Geometry check sheet. Reference: the model listing, model coordinates, mm. A direction names the side the tool comes from. Coordinates: 2 decimals unless noted, no trailing zeros. Write each loop counter-clockwise with the first axis right and the second up, starting at its lowest first coordinate (ties: lowest second). Pieces come first, ordered by that corner, then holes.
from build123d import *

# Parameters (mm, degrees)
F1_DEPTH = 3


with BuildPart() as f1:
    # F0 (on Front) → F1 (new body)
    with BuildSketch(Plane.XZ):
        with BuildLine():
            Line((-2.976018237, -3.4522186304), (-2.976018237, -0.7112144958))
            Line((-2.976018237, -0.7112144958), (-4.8061137058, 1.118880973))
            Line((-4.8061137058, 1.118880973), (-22.2056694329, 1.118880973))
            Line((-22.2056694329, 1.118880973), (-22.2056694329, -24.7238390148))
            ThreePointArc((-22.2056694329, -24.7238390148), (-12.5206211591, -30.5080748055), (-2.976018237, -24.494914338))
            Line((-2.976018237, -24.494914338), (-2.976018237, -5.1255999133))
            ThreePointArc((-2.976018237, -5.1255999133), (-3.0401081093, -4.2889092718), (-2.9760182369, -3.4522186304))
        make_face()
        with BuildLine():
            Line((-22.2056694329, 1.118880973), (-13.5058912988, 9.818658566))
            Line((-13.5058912988, 9.818658566), (-20.2551439519, 16.5679112191))
            ThreePointArc((-20.2551439519, 16.5679112191), (-21.4976121103, 14.4704948921), (-22.2056694329, 12.1377846226))
            Line((-22.2056694329, 12.1377846226), (-22.2056694329, 1.118880973))
        make_face()
        Polygon((-2.976018237, 3.3900048351), (-2.976018237, 20.348530973), (-11.4552815696, 11.8692681677), align=None)
        Polygon((-4.8061137058, 1.118880973), (-13.5058912988, 9.818658566), (-22.2056694329, 1.118880973), align=None)
        with BuildLine():
            Line((22.6377740155, 20.348530973), (-2.976018237, 20.348530973))
            Line((-2.976018237, 20.348530973), (-2.976018237, 3.3900048351))
            Line((-2.976018237, 3.3900048351), (-0.7048943749, 1.118880973))
            Line((-0.7048943749, 1.118880973), (1.486654611, 1.118880973))
            ThreePointArc((1.486654611, 1.118880973), (2.4534177425, 1.20461658), (3.4201808739, 1.118880973))
            Line((3.4201808739, 1.118880973), (27.0130801946, 1.118880973))
            ThreePointArc((27.0130801946, 1.118880973), (31.028528745, 12.1450925003), (22.6377740155, 20.348530973))
        make_face()
        with BuildLine():
            Line((-2.976018237, 20.348530973), (-14.1827978541, 20.348530973))
            ThreePointArc((-14.1827978541, 20.348530973), (-16.2761490838, 19.6875478868), (-18.179069268, 18.5930558661))
            Line((-18.179069268, 18.5930558661), (-11.4552815696, 11.8692681677))
            Line((-11.4552815696, 11.8692681677), (-2.976018237, 20.348530973))
        make_face()
        Polygon((-2.976018237, 1.118880973), (-2.976018237, 3.3900048351), (-11.4552815696, 11.8692681677), (-13.5058912988, 9.818658566), (-4.8061137058, 1.118880973), align=None)
        Polygon((-2.976018237, -0.7112144958), (-2.976018237, 1.118880973), (-4.8061137058, 1.118880973), align=None)
        with BuildLine():
            Line((-0.7048943749, 1.118880973), (-2.976018237, 1.118880973))
            Line((-2.976018237, 1.118880973), (-2.976018237, -0.7112144958))
            Line((-2.976018237, -0.7112144958), (-2.976018237, -3.4522186304))
            ThreePointArc((-2.9760182369, -3.4522186304), (-1.4774318683, -0.4512996484), (1.486654611, 1.118880973))
            Line((1.486654611, 1.118880973), (-0.7048943749, 1.118880973))
        make_face()
        Polygon((-0.7048943749, 1.118880973), (-2.976018237, 3.3900048351), (-2.976018237, 1.118880973), align=None)
        with BuildLine():
            Line((-2.976018237, -5.1255999133), (-2.976018237, -3.4522186304))
            ThreePointArc((-2.9760182369, -3.4522186304), (-3.0401081093, -4.2889092718), (-2.976018237, -5.1255999133))
        make_face()
        with BuildLine():
            ThreePointArc((3.4201808739, 1.118880973), (2.4534177425, 1.20461658), (1.486654611, 1.118880973))
            Line((1.486654611, 1.118880973), (3.4201808739, 1.118880973))
        make_face()
    extrude(amount=F1_DEPTH)


solid = f1.part
1. Thickness scan on line 1 along Z through (x, y) = (8.5, -2.45); line 2 along X through (y, z) = (-2.4, -13.5); line 3 along Z through (x, y) = (-12.5, -1.8). Record the ranges inside material, lowest first.
Computed values:
line 1: z = 1.12 to 20.35
line 2: x = -22.21 to -2.98
line 3: z = -30.51 to 10.82, 12.91 to 20.35
2. Gauge pin test, flat ends, axial feed: pin 1 Ø1.5 at (x, y) = (9, -1.5) entering from -Z; pin 2 Ø1 at (x, y) = (-14, -0.5) entering from -Z; pin 3 Ø0.9 at (y, z) = (-2, -16) entering from +X. Record the tip position at first contact, or that the pin passes through.
Computed values:
pin 1: stops at z = 1.12
pin 2: stops at z = -30.48
pin 3: stops at x = -2.98
3. Access from +Z, -Z, +X, -X, +Y, -Y to the whole of each face (thin tool, end or side, straight path). Record for faces 1 (the flat face through (-2.976, -1, -14)), 2 (the flat face through (-2, -3, 1)), 3 (the flat face through (-14.864, -1.479, 15.278)).
Computed values:
face 1: -Z, +X, +Y, -Y
face 2: +Z, -Z, +X, -X, -Y
face 3: +Y, -Y
4. Sectioned sample at C-C, the plane z = -11.5. Record the boundary of the cut face in (x, y).
Computed values:
outline: (-22.21, -3) - (-2.98, -3) - (-2.98, 0) - (-22.21, 0) - close
5. Sectioned sample at B-B, the plane x = 2.5. Record the boundary of the cut face in (y, z).
Computed values:
outline: (-3, 1.12) - (0, 1.12) - (0, 20.35) - (-3, 20.35) - close
6. Sectioned sample at A-A, the plane y = -1.75. Record the boundary of the cut face in (x, z).
Computed values:
outline: (-22.21, -24.72) arc R10.79 ccw to (-2.98, -24.49) - (-2.98, -3.45) arc R5.49 cw to (1.49, 1.12) - (27.01, 1.12) arc R10.82 ccw to (22.64, 20.35) - (-14.18, 20.35) arc R10.18 ccw to (-18.18, 18.59) - (-11.46, 11.87) - (-13.51, 9.82) - (-20.26, 16.57) arc R10.18 ccw to (-22.21, 12.14) - close
7. Draft check along X on faces 4 (the cylindrical face through (-12.69, -1.48, -30.51)), 5 (the cylindrical face through (-1.511, -1.479, -0.486)), 6 (the flat face through (-16.833, -1.479, 13.146)). Enter one of: released by +X, released by -X, zero draft, split by the parting line, or undercut.
Computed values:
face 4: split by the parting line
face 5: released by +X
face 6: undercut
